Build history of the part. All positions in model axes, mm. A direction names the side the tool comes from. Coordinates: 2 decimals unless noted, no trailing zeros. Order: outer loops, then holes, each group sorted by start corner. A loop starts at its lowest first (then second) coordinate and runs counter-clockwise, first axis right, second up. Notation, with made-up numbers: (-23.5, 57) - (1.5, 57) arc R16 cw to (1.5, 74) - close; hole circle Ø1 at (73.25, -22). An arc over 180 degrees is marked (long way). Write each question's results on one line, items separated by ' | '. Start each with the question number.
from build123d import *

# Parameters (mm, degrees)
SKETCH1_W           = 30
SKETCH1_H           = 45
BOSS_EXTRUDE1_DEPTH = 7.5
SKETCH2_R           = 12.5
CUT_EXTRUDE1_DEPTH  = 5.5
CUT_EXTRUDE2_REACH  = 4
SKETCH4_R           = 1.039999008
FILLET1_R           = 10
CUT_EXTRUDE3_REACH  = 9.5
SKETCH6_W           = 3.5
SKETCH6_H           = 34.5
SKETCH9_R           = 35
BOSS_EXTRUDE3_DEPTH = 7.5
CUT_EXTRUDE4_REACH  = 54.5
SKETCH10_R          = 9.525
SKETCH10_R_2        = 3.175


with BuildPart() as part:
    # Sketch1 → Boss-Extrude1 (new body)
    with BuildSketch(Plane.XY):
        Rectangle(SKETCH1_W, SKETCH1_H)
    extrude(amount=BOSS_EXTRUDE1_DEPTH)

    # Sketch2 → Cut-Extrude1 (cut)
    with BuildSketch(Plane.XY.offset(7.5)):
        with Locations((0, -7.5)):
            Circle(SKETCH2_R)
    extrude(amount=-CUT_EXTRUDE1_DEPTH, mode=Mode.SUBTRACT)

    # Sketch4 → Cut-Extrude2 (cut, up to next)
    with BuildSketch(Plane.XY.offset(2), mode=Mode.PRIVATE) as cut_extrude2_sk1:
        with Locations((0, -15.300000992)):
            Circle(SKETCH4_R)
    cut_extrude2_tool1 = extrude(cut_extrude2_sk1.sketch, amount=-CUT_EXTRUDE2_REACH, mode=Mode.PRIVATE) & part.part
    add(cut_extrude2_tool1.solids().sort_by_distance((0, -15.300001, 2))[0], mode=Mode.SUBTRACT)
    # Sketch4 → Cut-Extrude2 (cut, up to next)
    with BuildSketch(Plane.XY.offset(2), mode=Mode.PRIVATE) as cut_extrude2_sk2:
        with Locations((6.754999008, -3.599999504)):
            Circle(SKETCH4_R)
    cut_extrude2_tool2 = extrude(cut_extrude2_sk2.sketch, amount=-CUT_EXTRUDE2_REACH, mode=Mode.PRIVATE) & part.part
    add(cut_extrude2_tool2.solids().sort_by_distance((6.754999, -3.6, 2))[0], mode=Mode.SUBTRACT)
    # Sketch4 → Cut-Extrude2 (cut, up to next)
    with BuildSketch(Plane.XY.offset(2), mode=Mode.PRIVATE) as cut_extrude2_sk3:
        with Locations((-6.754999008, -3.599999504)):
            Circle(SKETCH4_R)
    cut_extrude2_tool3 = extrude(cut_extrude2_sk3.sketch, amount=-CUT_EXTRUDE2_REACH, mode=Mode.PRIVATE) & part.part
    add(cut_extrude2_tool3.solids().sort_by_distance((-6.754999, -3.6, 2))[0], mode=Mode.SUBTRACT)

    # Fillet1
    fillet1_edges = [part.edges().sort_by_distance(p)[0] for p in [
        (15, -22.5, 3.75),
        (-15, -22.5, 3.75),
    ]]
    fillet(fillet1_edges, radius=FILLET1_R)

    # Sketch6 → Cut-Extrude3 (cut, up to next)
    with BuildSketch(Plane.XY.offset(7.5), mode=Mode.PRIVATE) as cut_extrude3_sk1:
        with Locations((0, 9.75)):
            Rectangle(SKETCH6_W, SKETCH6_H)
    cut_extrude3_tool1 = extrude(cut_extrude3_sk1.sketch, amount=-CUT_EXTRUDE3_REACH, mode=Mode.PRIVATE) & part.part
    add(cut_extrude3_tool1.solids().sort_by_distance((0, 9.75, 7.5))[0], mode=Mode.SUBTRACT)

    # Sketch9 → Boss-Extrude3 (add)
    with BuildSketch(Plane(origin=(0, 22.5, 0), x_dir=(1, 0, 0), z_dir=(0, 1, 0))):
        with Locations((0, -22.449944321)):
            Circle(SKETCH9_R)
    extrude(amount=BOSS_EXTRUDE3_DEPTH)

    # Sketch10 → Cut-Extrude4 (cut, up to next)
    with BuildSketch(Plane(origin=(0, 30, 0), x_dir=(1, 0, 0), z_dir=(0, 1, 0)), mode=Mode.PRIVATE) as cut_extrude4_sk1:
        with Locations((0, -46.585066781)):
            Circle(SKETCH10_R)
    cut_extrude4_tool1 = extrude(cut_extrude4_sk1.sketch, amount=-CUT_EXTRUDE4_REACH, mode=Mode.PRIVATE) & part.part
    add(cut_extrude4_tool1.solids().sort_by_distance((0, 30, 46.585067))[0], mode=Mode.SUBTRACT)
    # Sketch10 → Cut-Extrude4 (cut, up to next)
    with BuildSketch(Plane(origin=(0, 30, 0), x_dir=(1, 0, 0), z_dir=(0, 1, 0)), mode=Mode.PRIVATE) as cut_extrude4_sk2:
        with Locations((-15.813770298, -18.629568863)):
            Circle(SKETCH10_R)
    cut_extrude4_tool2 = extrude(cut_extrude4_sk2.sketch, amount=-CUT_EXTRUDE4_REACH, mode=Mode.PRIVATE) & part.part
    add(cut_extrude4_tool2.solids().sort_by_distance((-15.81377, 30, 18.629569))[0], mode=Mode.SUBTRACT)
    # Sketch10 → Cut-Extrude4 (cut, up to next)
    with BuildSketch(Plane(origin=(0, 30, 0), x_dir=(1, 0, 0), z_dir=(0, 1, 0)), mode=Mode.PRIVATE) as cut_extrude4_sk3:
        with Locations((12.753899309, -11.844380068)):
            Circle(SKETCH10_R_2)
    cut_extrude4_tool3 = extrude(cut_extrude4_sk3.sketch, amount=-CUT_EXTRUDE4_REACH, mode=Mode.PRIVATE) & part.part
    add(cut_extrude4_tool3.solids().sort_by_distance((12.753899, 30, 11.84438))[0], mode=Mode.SUBTRACT)


solid = part.part
Item 1: Slice it at D-D (y = -3.6). Write the cut outline in (x, z) (3 decimals).
Item 2: Flat gauge pins, fed straight in: P1, Ø3, axis at x = 9.5, z = 37, coming from the -Y side; P2, Ø15, axis at x = 0, y = -7.5, coming from the -Z side; P3, Ø7.5, axis at x = -3.5, y = -2.5, coming from the +Z side. Where does each tip first touch, or does it go through?
Item 3: Pull direction Z, two halves, no side cores. Call faces 4 (the cylindrical face through (-2.065, 26.303, 55.884)), 5 (the flat face through (-4, 0, 0)), 6 (the cylindrical face through (-27.77, 26.2, 43.75)): released by +Z, released by -Z, zero draft, split by the parting line, or undercut.
Item 4: Slice it at C-C (z = 53.5). Write the cut outline in (x, y).
Item 5: Probe probe 1 along Y at (x, z) = (0, 1.6); probe 2 along X at (y, z) = (-7.5, 4.25); probe 3 along Y at (x, z) = (0, 3.25). List the from-to ranges inside material, lowest first.
Item 6: Slice it at A-A (y = 18). Write the cut outline in (x, z), then the cut area to 3 significant figures.
Item 7: Which spindle directions (+Z, -Z, +X, -X, +Y, -Y) get a long thin tool onto all of the face, cutting with end or side? Do faces 1 (the cylindrical face through (-0.53, -19.99, 4.79)), 2 (the flat face through (15, 5, 4)), 3 (the flat face through (-1.75, 11, 3)). Say none if no direction does.
Item 8: Slice it at B-B (x = 0). Write the cut outline in (y, z).
Resolved:
1) outline: (-15, 0) - (-7.795, 0) - (-7.795, 2) - (-11.876, 2) - (-11.876, 7.5) - (-15, 7.5) - close; (-5.715, 0) - (-1.75, 0) - (-1.75, 2) - (-5.715, 2) - close; (1.75, 0) - (5.715, 0) - (5.715, 2) - (1.75, 2) - close; (7.795, 0) - (15, 0) - (15, 7.5) - (11.876, 7.5) - (11.876, 2) - (7.795, 2) - close
2) P1: y = 22.5 | P2: z = 0 | P3: z = 2
3) face 4: undercut | face 5: released by -Z | face 6: split by the parting line
4) outline: (-16.15, 22.5) - (-6.55, 22.5) - (-6.55, 30) - (-16.15, 30) - close; (6.55, 22.5) - (16.15, 22.5) - (16.15, 30) - (6.55, 30) - close
5) probe 1: -22.5 to -16.34, -14.26 to -7.5, 22.5 to 30 | probe 2: -15 to -12.5, 12.5 to 15 | probe 3: -22.5 to -20, 22.5 to 30
6) outline: (-15, 0) - (-1.75, 0) - (-1.75, 7.5) - (-15, 7.5) - close; (1.75, 0) - (15, 0) - (15, 7.5) - (1.75, 7.5) - close | area: 199 mm^2
7) face 1: +Z | face 2: +Z, -Z, +X, -Y | face 3: +Z, -Z
8) outline: (-22.5, 0) - (-16.34, 0) - (-16.34, 2) - (-20, 2) - (-20, 7.5) - (-22.5, 7.5) - close; (-14.26, 0) - (-7.5, 0) - (-7.5, 2) - (-14.26, 2) - close; (22.5, -12.55) - (30, -12.55) - (30, 37.06) - (22.5, 37.06) - close; (22.5, 56.11) - (30, 56.11) - (30, 57.45) - (22.5, 57.45) - close
